Study the drawing (mm; zero at the part's minimum x, y, z) and answer. A direction names the side the tool comes from. Give positions to 0.01 mm unless a question says otherwise; leave off trailing zeros. Loops run counter-clockwise (first coordinate to the right, second up) from the corner with the lowest first, then second, coordinate; pieces in that order, holes last. Notation, with made-up numbers: M 78.5,-1 L 121.5,-1 A21 cw 121.5,14 Z; hole C 84,-27.75 d6. An arc over 180 degrees is marked long. Return JSON: item names as keys, results as strings.
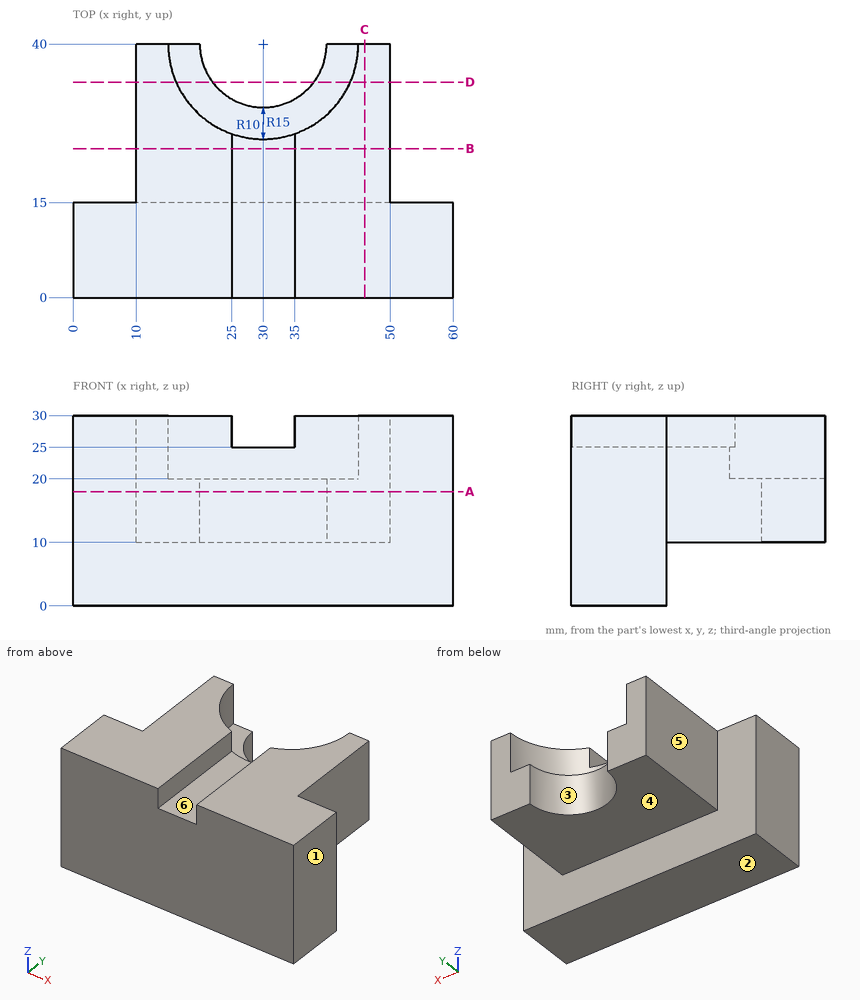
(1) The part is cut by section D-D (y = 34). Determine the outline of the cut face in (x, z).
Values follow:
{"outline": "M 10,10 L 22,10 L 22,20 L 16.25,20 L 16.25,30 L 10,30 Z; M 38,10 L 50,10 L 50,30 L 43.75,30 L 43.75,20 L 38,20 Z"}
(2) Determine the mould class of the marked faces 1, 2 and 3 for opening direction X: released by +X, released by -X, zero draft, split by the parting line, or undercut.
Values follow:
{"face 1": "released by +X", "face 2": "zero draft", "face 3": "undercut"}
(3) The part is cut by section C-C (x = 46). Determine the outline of the cut face in (y, z).
Values follow:
{"outline": "M 0,0 L 15,0 L 15,10 L 40,10 L 40,30 L 0,30 Z"}
(4) Given pin 1 (3 mm diameter, centred on x = 29, y = 7, fed in from +Z); pin 2 (1 mm diameter, centred on y = 28, z = 18, fed in from +X); pin 3 (6 mm diameter, centred on x = 29.5, z = 10.5, fed in from +Y), each flat-ended and moving along its own axis, determine where each tip first touches the part or whether it passes through.
Values follow:
{"pin 1": "z = 25", "pin 2": "x = 50", "pin 3": "y = 30.63"}
(5) Straight lines are drawn through the part: line 1 along X through (y, z) = (19, 28.5); line 2 along Y through (x, z) = (43.5, 3); line 3 along Z through (x, y) = (38, 17.5). For each, find the intervals that lie inside material, in ascending order.
Values follow:
{"line 1": "10 to 25, 35 to 50", "line 2": "0 to 15", "line 3": "10 to 30"}
(6) The part is cut by section B-B (y = 23.5). Determine the outline of the cut face in (x, z).
Values follow:
{"outline": "M 10,10 L 50,10 L 50,30 L 35,30 L 35,25 L 25,25 L 25,30 L 10,30 Z"}
(7) A tool of negligible diameter and unlimited length cuts with its end or side. For the marked faces 4, 5 and 6, from which of +Z, -Z, +X, -X, +Y, -Y can it reach the whole face along a straight path? Write none if from no direction.
Values follow:
{"face 4": "-Z, +X, -X, +Y", "face 5": "+Z, -Z, -X, +Y", "face 6": "+Z, +Y, -Y"}
(8) The part is cut by section A-A (z = 18). Determine the outline of the cut face in (x, y), and give its area (3 significant figures).
Values follow:
{"outline": "M 0,0 L 60,0 L 60,15 L 50,15 L 50,40 L 40,40 A10 cw 20,40 L 10,40 L 10,15 L 0,15 Z", "area": "1,740 mm²"}
